Autodesk Inventor part; units mm, degrees
ref_plane "YZ Plane" through (0, 0, 0) normal (1, 0, 0) x (0, 1, 0)
ref_plane "XZ Plane" through (0, 0, 0) normal (0, 1, 0) x (-1, 0, 0)
ref_plane "XY Plane" through (0, 0, 0) normal (0, 0, 1) x (1, 0, 0)
sketch "Boceto1" plane through (0, 0, 0) normal (0, 0, 1) x (1, 0, 0)
  line L0 (19, -10.5) -> (-20.5, -10.5)
  arc A0 (19, -10.5) -> (20.5, -9) centre (19, -9) ccw
  line L1 (20.5, 9) -> (20.5, -9)
  arc A1 (20.5, 9) -> (19, 10.5) centre (19, 9) ccw
  line L2 (-20.5, 10.5) -> (19, 10.5)
  line L3 (-20.5, -10.5) -> (-20.5, 10.5)
  line L4 (-21, -11) -> (19, -11)
  arc A2 (19, -11) -> (21, -9) centre (19, -9) ccw
  line L5 (21, -9) -> (21, 9)
  arc A3 (21, 9) -> (19, 11) centre (19, 9) ccw
  line L6 (19, 11) -> (-21, 11)
  line L7 (-21, 11) -> (-21, -11)
  spline S0 degree 3 poles (-19.1456, -15) (-19.0838, -15) (-18.9941, -14.9843) (-18.7809, -14.9428) (-18.6401, -14.9132) (-18.3299, -14.8682) (-18.1603, -14.854) (-18, -14.854) (-17.8397, -14.854) (-17.6701, -14.8682) (-17.3599, -14.9132) (-17.2191, -14.9428) (-17.0059, -14.9843) (-16.9162, -15) (-16.8544, -15) knots 0.670558 0.670558 0.670558 0.670558 0.714606 0.714606 0.762709 0.762709 0.810813 0.810813 0.810813 0.858917 0.858917 0.907021 0.907021 0.951069 0.951069 0.951069 0.951069
  line L8 (-16.75, -15) -> (-19.25, -15)
  line L9 (-16.75, -15) -> (-19.25, -15)
  spline S1 degree 3 poles (-19.1456, -15) (-19.0838, -15) (-18.9941, -14.9843) (-18.7809, -14.9428) (-18.6401, -14.9132) (-18.3299, -14.8682) (-18.1603, -14.854) (-18, -14.854) (-17.8397, -14.854) (-17.6701, -14.8682) (-17.3599, -14.9132) (-17.2191, -14.9428) (-17.0059, -14.9843) (-16.9162, -15) (-16.8544, -15) knots 0.670558 0.670558 0.670558 0.670558 0.714606 0.714606 0.762709 0.762709 0.810813 0.810813 0.810813 0.858917 0.858917 0.907021 0.907021 0.951069 0.951069 0.951069 0.951069
  line L10 (-16.75, -15) -> (-19.25, -15)
  line L11 (-18, -15) -> (-18, 10.5)
  line L12 (-18, -10.5) -> (-20, -10.5)
  line L13 (-20, -10.5) -> (-20, 10.5)
  arc A4 (20, 9) -> (19, 10) centre (19, 9) ccw
  line L14 (20, 9) -> (20, -9)
  arc A5 (19, -10) -> (20, -9) centre (19, -9) ccw
  line L15 (19, -10) -> (-20, -10)
  line L16 (-20, -10) -> (-20, 10)
  line L17 (-20, 10) -> (19, 10)
  point P0 (0, 0)
  point P1 (-18, 10)
  point P2 (-20, 10)
  dimension "d0" = 0.5
  dimension "d1" = 2
  dimension "d25" = 0.5
extrude "Extrusión1" add sketch "Boceto1" along normal blind 5 contours L15 L13 L17 L11 | L11 L17 A4 L14 A5 L15
fillet "Empalme1" radius 2.5 2 edges at (-20, 0, 5) (-20, 0, 0)
sketch "Boceto4" plane through (0, 0, 5) normal (0, 0, 1) x (1, 0, 0)
  line L0 (-17.5, -10) -> (-17.5, 10)
  line L1 (18.5, 10.5) -> (19, 10.5)
  line L2 (18.5, 10.5) -> (18.5, -10.5)
  line L3 (19, -10.5) -> (18.5, -10.5)
  line L4 (18.5, -10.5) -> (19, -10.5)
  line L5 (18.5, 10.5) -> (18.5, -10.5)
  line L6 (19, 10.5) -> (18.5, 10.5)
  line L7 (20.5, 9) -> (20.5, -9)
  line L8 (25.5, -7.5) -> (19, -7.5)
  line L9 (15.5, -4) -> (15.5, 4)
  line L10 (19, 7.5) -> (25.5, 7.5)
  line L11 (25.5, 7.5) -> (25.5, -7.5)
  line L12 (25.5, -7.5) -> (15.5, 7.5) construction
  line L13 (15.5, -7.5) -> (25.5, 7.5) construction
  arc A0 (19, 7.5) -> (15.5, 4) centre (19, 4) ccw
  arc A1 (15.5, -4) -> (19, -7.5) centre (19, -4) ccw
  line L14 (-17.5, -10) -> (19, -10)
  arc A2 (19, -10) -> (20, -9) centre (19, -9) ccw
  line L15 (20, -9) -> (20, 9)
  arc A3 (20, 9) -> (19, 10) centre (19, 9) ccw
  line L16 (19, 10) -> (-17.5, 10)
  point P0 (0, 0)
  point P1 (20.5, 0)
  point P2 (20.5, -7.5)
  point P3 (20.5, 7.5)
  point P4 (18.5, -7.4641)
  point P5 (18.5, 7.4641)
  point P6 (20, -7.5)
  point P7 (18.5, -10)
  point P8 (20.5, 7.5)
  point P9 (20.5, -7.5)
  point P10 (18.5, 10)
  point P11 (20, 7.5)
  point P12 (20, 7.5)
  point P13 (20, -7.5)
  dimension "d15" = 10
  dimension "d16" = 15
  dimension "d17" = 3.5
extrude "Extrusión3" cut sketch "Boceto4" against normal blind 10 contours A1 L9 A0 L2 | L2 A0 L10 L15 L8 A1 | L15 L10 L7 L8 | L7 L10 L11 L8
sketch "Boceto6" plane through (19, -10, 0) normal (0, -1, 0) x (1, 0, 0)
  arc A0 (-36.5, 5) -> (-36.5, 0) centre (-36.5, 2.5) ccw
  point P0 (-19, 0)
  point P1 (-39, 3)
hole "Agujero2" at (-17.5, -10, 2.5) direction (0, 1, 0) diameter 2.5 end through all
properties part number "Brazo2_2"
Work out the finished part from the listing and answer in its coordinate system (mm). A direction names the side the tool comes from. Give positions to 0.01 mm unless a question says otherwise; leave off trailing zeros. Loops run counter-clockwise (first coordinate to the right, second up) from the corner with the lowest first, then second, coordinate; pieces in that order, holes last. Notation, with made-up numbers: (-39.75, 1.5) -> (8.25, 1.5) arc R19 cw to (8.25, 29.5) -> close; hole circle Ø7 at (19, 39.5). An arc over 180 degrees is marked (long way). Use a Markdown table: item, result. Add a question column.
1) The part is cut by section A-A, the plane x = 17. Determine the outline of the cut face in (y, z), plus the area to 3 significant figures.
2) For a pull along Y with two mould halves and no side action, classify faces 3 (the cylindrical face through (-19.287, 0.14, 4.248)), 4 (the cylindrical face through (19.699, 9.715, 2.465)), 5 (the flat face through (19.5, -7.5, 2.5)) as +Y half, -Y half, draft (parallel to the pull), parting line (faces both ways), or undercut.
3) Which of the six approach directions +Z, -Z, +X, -X, +Y, -Y give full straight-line access (tool end or side, diameter ignored) to faces 1 (the flat face through (19.5, 7.5, 2.5)), 2 (the flat face through (0, -10, 2))?
4) Consider line 1 along X through (y, z) = (3.75, 2.5); line 2 along Z through (x, y) = (-17.5, -3); line 3 along Y through (x, z) = (16.5, 2.35). Determine where each line is inside the solid, lowest interval first.
5) Each of these flat-tipped pins is pushed along its axis until it touches: P1, Ø2.5, axis at y = 1, z = 2, coming from the +X side; P2, Ø2, axis at x = -17.5, z = 2.5, coming from the -Y side; P3, Ø0.8, axis at x = 19.5, z = 1.5, coming from the -Y side (3 decimals). Where does it stop, or does it pass through?
Reported:
| question | item | result |
|---|---|---|
| 1 | outline | (-10, 0) -> (-6.87, 0) -> (-6.87, 5) -> (-10, 5) -> close; (6.87, 0) -> (10, 0) -> (10, 5) -> (6.87, 5) -> close |
| 1 | area | 31.3 mm^2 |
| 2 | face 3 | draft |
| 2 | face 4 | +Y half |
| 2 | face 5 | undercut |
| 3 | face 1 | +Z, -Z, +X |
| 3 | face 2 | +Z, -Z, +X, -X, -Y |
| 4 | line 1 | x = -20 to -18.75, -16.25 to 15.5 |
| 4 | line 2 | z = 0 to 1.25, 3.75 to 5 |
| 4 | line 3 | y = -10 to -6.45, 6.45 to 10 |
| 5 | P1 | stops at x = 15.5 |
| 5 | P2 | passes through |
| 5 | P3 | stops at y = -9.995 |
